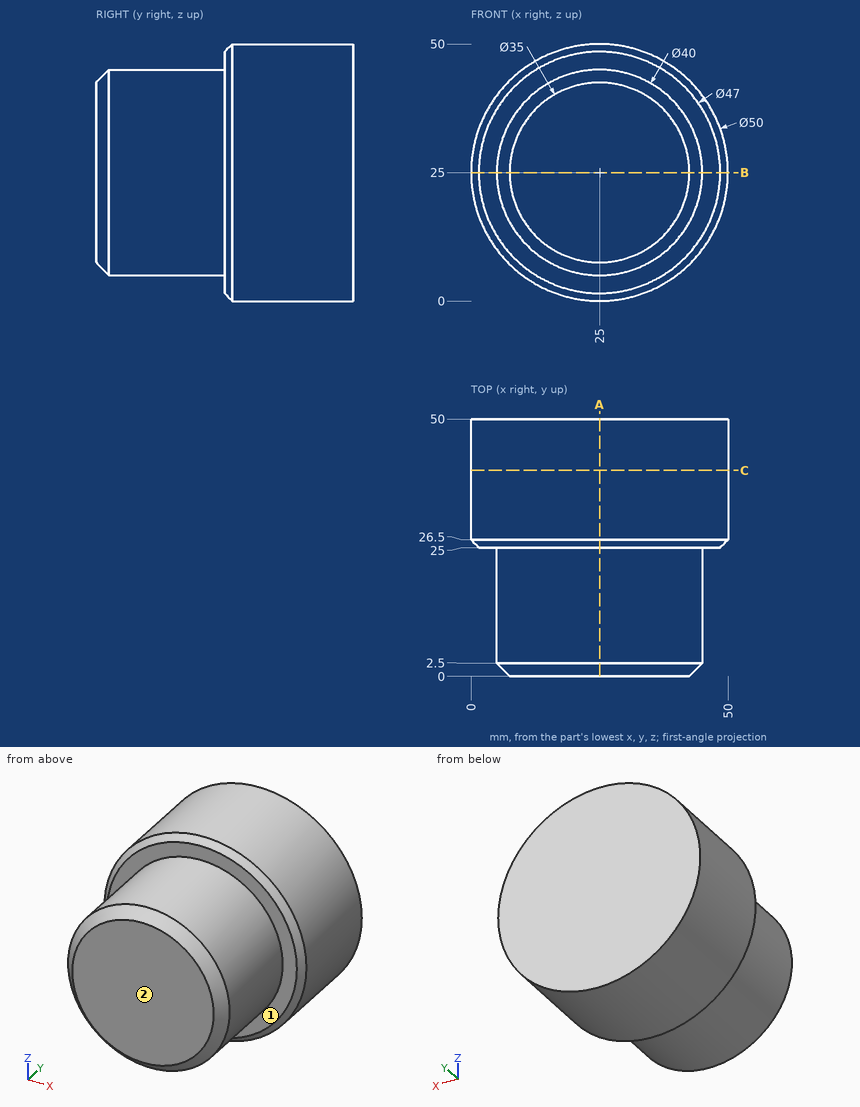
Input: dimensioned drawing with shaded views. Units: mm. Origin: part minimum x, y, z. A direction names the side the tool comes from. Give positions to 0.01 mm unless a question says otherwise; leave off trailing zeros. Order: outer loops, then holes, each group sorted by start corner. A loop starts at its lowest first (then second) coordinate and runs counter-clockwise, first axis right, second up.
(1) Access query for the marked faces 1 and 2. Directions: +Z, -Z, +X, -X, +Y, -Y. A direction counts if a zero-diameter tool reaches every point of the face in a straight line with its end or side. Return the directions, or none.
(2) Section query B-B (z = 25). Return the cut outline in (x, y), plus the area to 3 significant figures.
(3) Contact query for flat-ended pins moving along their axis: P1, Ø3, axis at x = 32.5, y = 28, coming from the +Z side; P2, Ø2, axis at y = 8, z = 9, coming from the -X side; P3, Ø1.5, axis at x = 44, y = 40, coming from the +Z side. Output: stop coordinate, or through.
(4) Section query A-A (x = 25). Return the cut outline in (y, z).
(5) Material intervals for line 1 along Y through (x, z) = (20, 5); line 2 along X through (y, z) = (33, 25.5) (3 decimals); line 3 along Z through (x, y) = (2, 30.5), sorted ascending.
(6) Section query C-C (y = 40). Return the cut outline in (x, z), plus the area to 3 significant figures.
Outcome:
1. face 1: -Y
1. face 2: +Z, -Z, +X, -X, -Y
2. outline: (0, 26.5) - (1.5, 25) - (5, 25) - (5, 2.5) - (7.5, 0) - (42.5, 0) - (45, 2.5) - (45, 25) - (48.5, 25) - (50, 26.5) - (50, 50) - (0, 50) - close
2. area: 2,240 mm2
3. P1: stops at z = 49.27
3. P2: stops at x = 11.77
3. P3: stops at z = 42.09
4. outline: (0, 7.5) - (2.5, 5) - (25, 5) - (25, 1.5) - (26.5, 0) - (50, 0) - (50, 50) - (26.5, 50) - (25, 48.5) - (25, 45) - (2.5, 45) - (0, 42.5) - close
5. line 1: y = 25 to 50
5. line 2: x = 0.005 to 49.995
5. line 3: z = 15.2 to 34.8
6. outline: circle Ø50 at (25, 25)
6. area: 1,960 mm2
